Autodesk Inventor part; units mm, degrees
ref_plane "YZ Plane" through (0, 0, 0) normal (1, 0, 0) x (0, 1, 0)
ref_plane "XZ Plane" through (0, 0, 0) normal (0, 1, 0) x (-1, 0, 0)
ref_plane "XY Plane" through (0, 0, 0) normal (0, 0, 1) x (1, 0, 0)
sketch "Sketch1" plane through (0, 0, 0) normal (0, 1, 0) x (-1, 0, 0)
  line L0 (-19.05, -19.05) -> (19.05, -19.05)
  line L1 (19.05, -19.05) -> (19.05, 19.05)
  line L2 (19.05, 19.05) -> (-19.05, 19.05)
  line L3 (-19.05, 19.05) -> (-19.05, -19.05)
  line L4 (-19.05, -19.05) -> (19.05, 19.05) construction
  line L5 (19.05, -19.05) -> (-19.05, 19.05) construction
  point P0 (0, 0)
  dimension "d0" = 38.1
  dimension "d1" = 38.1
extrude "Extrusion1" add sketch "Sketch1" along normal blind 2.54
sketch "Sketch2" plane through (0, 2.54, 0) normal (0, 1, 0) x (1, 0, 0)
  line L0 (13.97, -2.54) -> (-13.97, -2.54)
  line L1 (-13.97, -2.54) -> (-13.97, 2.54)
  line L2 (-13.97, 2.54) -> (13.97, 2.54)
  line L3 (13.97, 2.54) -> (13.97, -2.54)
  line L4 (-19.05, 19.05) -> (-19.05, -19.05)
  line L5 (19.05, -19.05) -> (19.05, 19.05)
  line L6 (19.05, 19.05) -> (-19.05, 19.05)
  point P0 (0, 0)
  dimension "d4" = 5.08
  dimension "d5" = 5.08
  dimension "d6" = 16.51
  dimension "d7" = 5.08
extrude "Extrusion2" add sketch "Sketch2" along normal blind 25.4
sketch "Sketch3" plane through (-13.97, 2.54, 2.54) normal (0, 0, 1) x (1, 0, 0)
  circle A0 centre (13.97, 15.5704) radius 8.0645
  point P0 (13.97, -2.54)
  dimension "d10" = 16.129
extrude "Extrusion3" cut sketch "Sketch3" against normal blind 50.8
sketch "Sketch4" plane through (0, 2.54, 0) normal (0, 1, 0) x (1, 0, 0)
  circle A0 centre (-12.7, -12.7) radius 2.5797
  circle A1 centre (-12.7, 12.7) radius 2.5797
  circle A2 centre (12.7, 12.7) radius 2.5797
  circle A3 centre (12.7, -12.7) radius 2.5797
  line L0 (-19.05, 19.05) -> (-19.05, -19.05)
  line L1 (-19.05, -19.05) -> (19.05, -19.05)
  line L2 (19.05, -19.05) -> (19.05, 19.05)
  line L3 (19.05, 19.05) -> (-19.05, 19.05)
  point P0 (0, 0)
  dimension "d13" = 5.1594
  dimension "d14" = 5.1594
  dimension "d15" = 5.1594
  dimension "d16" = 5.1594
  dimension "d17" = 6.35
  dimension "d18" = 6.35
  dimension "d19" = 6.35
  dimension "d20" = 6.35
  dimension "d21" = 6.35
  dimension "d22" = 6.35
  dimension "d23" = 6.35
  dimension "d24" = 6.35
extrude "Extrusion4" cut sketch "Sketch4" against normal blind 50.8 contours A0 | A1 | A2 | A3
equation "\"d1\" = d0"
equation "\"d4\" = d5"
equation "\"d14\" = d13"
equation "\"d15\" = d13"
equation "\"d16\" = d13"
equation "\"d18\" = d17"
equation "\"d19\" = d17"
equation "\"d20\" = d17"
equation "\"d21\" = d17"
equation "\"d22\" = d17"
equation "\"d23\" = d17"
equation "\"d24\" = d17"
properties part number "pneumatics front holder"
Work out the finished part from the listing and answer in its coordinate system (mm). A direction names the side the tool comes from. Coordinates: 2 decimals unless noted, no trailing zeros. Write each loop counter-clockwise with the first axis right and the second up, starting at its lowest first coordinate (ties: lowest second). Pieces come first, ordered by that corner, then holes. Notation, with made-up numbers: M -11,30 L -4,30 A18 ccw -4,43 Z; hole C 33.5,46.25 d6. An arc over 180 degrees is marked long. Write item = value, one per line.
1. Flat-ended cylindrical pins translate along their axes: pin 1 (12 mm diameter, centred on y = 13.5, z = -13, fed in from -X); pin 2 (8 mm diameter, centred on x = -9, y = 12.5, fed in from +Z); pin 3 (8.5 mm diameter, centred on x = -12.7, z = 12.7, fed in from +Y); pin 4 (3 mm diameter, centred on y = 13.5, z = 0, fed in from +X). Find the tip coordinate at first contact, or state that the pin passes through.
Solution:
pin_1 = through
pin_2 = 2.54
pin_3 = 2.54
pin_4 = 13.97
2. Straight lines are drawn through the part: line 1 (X direction, y = 1.2, z = 12.7); line 2 (Y direction, x = 0, z = 0.65). For each, find the intervals that lie inside material, in ascending order. Write a range as from..to.
Solution:
line_1 = -19.05..-15.28, -10.12..10.12, 15.28..19.05
line_2 = 0..10.05, 26.17..27.94
3. The part is cut by section D-D (y = 24.75). Determine the outline of the cut face in (x, z), then the cut area to 3 significant figures.
Solution:
outline = M -13.97,-2.54 L -4.58,-2.54 L -4.58,2.54 L -13.97,2.54 Z; M 4.58,-2.54 L 13.97,-2.54 L 13.97,2.54 L 4.58,2.54 Z
area = 95.4 mm2
4. The part is cut by section A-A (x = 0). Determine the outline of the cut face in (y, z), then the cut area to 3 significant figures.
Solution:
outline = M 0,-19.05 L 2.54,-19.05 L 2.54,-2.54 L 10.05,-2.54 L 10.05,2.54 L 2.54,2.54 L 2.54,19.05 L 0,19.05 Z; M 26.17,-2.54 L 27.94,-2.54 L 27.94,2.54 L 26.17,2.54 Z
area = 144 mm2
5. The part is cut by section B-B (z = 12.7). Determine the outline of the cut face in (x, y).
Solution:
outline = M -19.05,0 L -15.28,0 L -15.28,2.54 L -19.05,2.54 Z; M -10.12,0 L 10.12,0 L 10.12,2.54 L -10.12,2.54 Z; M 15.28,0 L 19.05,0 L 19.05,2.54 L 15.28,2.54 Z
6. Determine the mould class of faces 6 (the face through (14.087, 1.288, 10.525)), 7 (the face through (0, 27.94, 0)), 8 (the face through (3.721, 10.956, 0.036)) for opening direction Y: released by +Y, released by -Y, zero draft, split by the parting line, or undercut.
Solution:
face_6 = zero draft
face_7 = released by +Y
face_8 = undercut
7. For faces 1 (the face through (-13.97, 15, 0)), 2 (the face through (13.97, 15, 0)), 3 (the face through (-19.05, 1, 0)), 4 (the face through (0, 9, -2.54)), 5 (the face through (0, 9, 2.54)), determine the directions among +Z, -Z, +X, -X, +Y, -Y from which every point of the face is accessible in a straight line to the end or side of a thin tool.
Solution:
face_1 = +Z, -Z, -X, +Y
face_2 = +Z, -Z, +X, +Y
face_3 = +Z, -Z, -X, +Y, -Y
face_4 = -Z, +X, -X, +Y
face_5 = +Z, +X, -X, +Y
8. The part is cut by section C-C (x = 12.7). Determine the outline of the cut face in (y, z).
Solution:
outline = M 0,-19.05 L 2.54,-19.05 L 2.54,-15.28 L 0,-15.28 Z; M 0,-10.12 L 2.54,-10.12 L 2.54,-2.54 L 27.94,-2.54 L 27.94,2.54 L 2.54,2.54 L 2.54,10.12 L 0,10.12 Z; M 0,15.28 L 2.54,15.28 L 2.54,19.05 L 0,19.05 Z
